For this review, take the finished solid that the model builds, in its own axes (mm). A direction names the side the tool comes from. Give positions to 0.01 mm unless a question says otherwise; leave off trailing zeros. Write each loop counter-clockwise with the first axis right and the second up, starting at its lowest first coordinate (ties: lowest second). Pieces come first, ordered by that corner, then holes. Notation, with made-up numbers: (44, 3.5) -> (51, 3.5) arc R18 cw to (51, 36.5) -> close; hole circle Ø1 at (-7.75, -17.75). An arc over 180 degrees is marked (long way). Return JSON: item names as keys, results as strings.
from build123d import *

# Parameters (mm, degrees)
BOSS_EXTRUDE1_DEPTH = 6
SKETCH2_R           = 1.35
CUT_EXTRUDE1_DEPTH  = 30.086079144


with BuildPart() as part:
    # Sketch1 → Boss-Extrude1 (new body)
    with BuildSketch(Plane(origin=(0, 0, 0), x_dir=(1, 0, 0), z_dir=(0, 1, 0))):
        Polygon((-5.5, 2.5), (-5.5, 9), (-16.5, 9), (-16.5, 6), (-10.5, 6), (-10.5, 1.847803827), (-10.5, 0), (-10.5, -6), (-16.5, -6), (-16.5, -9), (-5.5, -9), (-5.5, -2.5), (5.5, -2.5), (5.5, -9), (10.5, -9), (13.5, -9), (13.5, -6), (10.5, -6), (10.5, 0), (10.5, 6), (13.5, 6), (13.5, 9), (10.5, 9), (5.5, 9), (5.5, 2.5), align=None)
    extrude(amount=BOSS_EXTRUDE1_DEPTH)

    # Sketch2 → Cut-Extrude1 (cut, through all)
    with BuildSketch(Plane(origin=(10.5, 0, 0), x_dir=(0, 0, -1), z_dir=(1, 0, 0))):
        with Locations((0, 3)):
            Circle(SKETCH2_R)
    extrude(amount=-CUT_EXTRUDE1_DEPTH, mode=Mode.SUBTRACT)


solid = part.part
1. For pin 1 (3 mm diameter, centred on y = 3, z = 0, fed in from -X); pin 2 (3 mm diameter, centred on y = 1.5, z = -5.5, fed in from +X); pin 3 (3 mm diameter, centred on y = 3.5, z = 1, fed in from +X); pin 4 (3 mm diameter, centred on x = 0, y = 4, fed in from -Z), all flat-tipped, find the tip position at first contact; note any pin that passes through.
Results found:
{"pin 1": "stops at x = -10.5", "pin 2": "stops at x = 13.5", "pin 3": "stops at x = 10.5", "pin 4": "stops at z = -2.5"}
2. To check wall thickness, follow probe 1 along Z at (x, y) = (-13.25, 3.85); probe 2 along X at (y, z) = (4.8, 7.5); probe 3 along Y at (x, z) = (-0.5, 0). State the ranges of each line that lie inside material, in increasing order.
Results found:
{"probe 1": "z = -9 to -6, 6 to 9", "probe 2": "x = -16.5 to -5.5, 5.5 to 13.5", "probe 3": "y = 0 to 1.65, 4.35 to 6"}
3. For faces 5 (the flat face through (-5.5, 3, 6)), 6 (the flat face through (12, 3, 6)), 7 (the flat face through (0, 3, -2.5)), 8 (the flat face through (13.5, 3, 8)), 9 (the flat face through (-14, 3, -6)), list the 3-axis set-ups (+Z, -Z, +X, -X, +Y, -Y) from which the entire face can be reached by the end or side of a thin tool; tool diameter is ignored.
Results found:
{"face 5": "+Z, +Y, -Y", "face 6": "+X, +Y, -Y", "face 7": "-Z, +Y, -Y", "face 8": "+Z, -Z, +X, +Y, -Y", "face 9": "-X, +Y, -Y"}
4. Add section D-D, the plane y = 1.2. State the section outline as (x, z) points, plus the area to 3 significant figures.
Results found:
{"outline": "(-16.5, -9) -> (-5.5, -9) -> (-5.5, -2.5) -> (5.5, -2.5) -> (5.5, -9) -> (13.5, -9) -> (13.5, -6) -> (10.5, -6) -> (10.5, 6) -> (13.5, 6) -> (13.5, 9) -> (5.5, 9) -> (5.5, 2.5) -> (-5.5, 2.5) -> (-5.5, 9) -> (-16.5, 9) -> (-16.5, 6) -> (-10.5, 6) -> (-10.5, -6) -> (-16.5, -6) -> close", "area": "289 mm²"}
5. Add section B-B, the plane y = 3. State the section outline as (x, z) points.
Results found:
{"outline": "(-16.5, -9) -> (-5.5, -9) -> (-5.5, -2.5) -> (5.5, -2.5) -> (5.5, -9) -> (13.5, -9) -> (13.5, -6) -> (10.5, -6) -> (10.5, -1.35) -> (-10.5, -1.35) -> (-10.5, -6) -> (-16.5, -6) -> close; (-16.5, 6) -> (-10.5, 6) -> (-10.5, 1.35) -> (10.5, 1.35) -> (10.5, 6) -> (13.5, 6) -> (13.5, 9) -> (5.5, 9) -> (5.5, 2.5) -> (-5.5, 2.5) -> (-5.5, 9) -> (-16.5, 9) -> close"}
6. Add section A-A, the plane z = -6.5. State the section outline as (x, y) points, plus the area to 3 significant figures.
Results found:
{"outline": "(-16.5, 0) -> (-5.5, 0) -> (-5.5, 6) -> (-16.5, 6) -> close; (5.5, 0) -> (13.5, 0) -> (13.5, 6) -> (5.5, 6) -> close", "area": "114 mm²"}
7. The part is to be moulded in two halves that separate along Y. For faces 1 (the cylindrical face through (0.15, 1.68, 0.29)), 2 (the flat face through (5.5, 3, -6)), 3 (the flat face through (-2, 6, 0)), 4 (the flat face through (-2, 0, 0)), say which applies: +Y half, -Y half, draft (parallel to the pull), parting line (faces both ways), or undercut.
Results found:
{"face 1": "undercut", "face 2": "draft", "face 3": "+Y half", "face 4": "-Y half"}
8. Add section C-C, the plane x = 4.5. State the section outline as (y, z) points.
Results found:
{"outline": "(0, -2.5) -> (6, -2.5) -> (6, 2.5) -> (0, 2.5) -> close; hole circle Ø2.7 at (3, 0)"}
